```python
from build123d import *

# Parameters (mm, degrees)
F0_R           = 1.0414
F1_DEPTH       = 12.7
F3_D           = 2.0828
F3_CBORE_D     = 6.858
F3_CBORE_DEPTH = 4.1656


with BuildPart() as f1:
    # F0 (on Top) → F1 (new body)
    with BuildSketch(Plane.XY):
        with BuildLine():
            ThreePointArc((-68.834, -13.75156), (-68.090051, -15.547611), (-66.294, -16.29156))
            Line((-66.294, -16.29156), (66.294, -16.29156))
            ThreePointArc((66.294, -16.29156), (68.090051, -15.547611), (68.834, -13.75156))
            Line((68.834, -13.75156), (68.834, 13.75156))
            ThreePointArc((68.834, 13.75156), (68.090051, 15.547611), (66.294, 16.29156))
            Line((66.294, 16.29156), (-66.294, 16.29156))
            ThreePointArc((-66.294, 16.29156), (-68.090051, 15.547611), (-68.834, 13.75156))
            Line((-68.834, 13.75156), (-68.834, -13.75156))
        make_face()
        with Locations((-65.278, -10.16)):
            Circle(F0_R, mode=Mode.SUBTRACT)
        with Locations((65.278, -10.16)):
            Circle(F0_R, mode=Mode.SUBTRACT)
        with Locations((-65.278, 10.16)):
            Circle(F0_R, mode=Mode.SUBTRACT)
        with Locations((65.278, 10.16)):
            Circle(F0_R, mode=Mode.SUBTRACT)
    extrude(amount=F1_DEPTH)

    # F3 (through all)
    with Locations(Plane(origin=(0, 0, 0), x_dir=(1, 0, 0), z_dir=(0, 0, -1))):
        with Locations((-35.56, 5.08), (-35.56, -5.08)):
            CounterBoreHole(F3_D / 2, F3_CBORE_D / 2, F3_CBORE_DEPTH)


solid = f1.part
```
Could you check a few things on this model? Use its own coordinates, in mm. A direction names the side the tool comes from. Coordinates: 2 decimals unless noted, no trailing zeros. Write each loop counter-clockwise with the first axis right and the second up, starting at its lowest first coordinate (ties: lowest second). Pieces come first, ordered by that corner, then holes. Notation, with made-up numbers: (18, 77.5) - (36, 77.5) arc R8 cw to (36, 90.5) - close; hole circle Ø9 at (-34.5, -38.5). An arc over 180 degrees is marked (long way). Use a Markdown table: item, result.
Q1. Which directions (+Z, -Z, +X, -X, +Y, -Y) give clear straight access to the entire face, cutting with the end or side of a thin tool? Please do faces 1 (the cylindrical face through (68.07, -15.57, 6.26)), 2 (the flat face through (-35.6, -3.6, 4.166)).
Geometry check:
| item | result |
|---|---|
| face 1 | +Z, -Z, +X, -Y |
| face 2 | -Z |
Q2. Please list where these lines run through material, in increasing order: L1, parallel to Y at x = -35.56, z = 10.5; L2, parallel to X at y = -10, z = 8; L3, parallel to Y at x = -35.56, z = 1.9.
Geometry check:
| item | result |
|---|---|
| L1 | y = -16.29 to -6.12, -4.04 to 4.04, 6.12 to 16.29 |
| L2 | x = -68.83 to -66.31, -64.25 to 64.25, 66.31 to 68.83 |
| L3 | y = -16.29 to -8.51, -1.65 to 1.65, 8.51 to 16.29 |
Q3. I'm going to push flat-ended pins straight in: pin 1 Ø11 at (x, y) = (-35.56, -5.08) entering from -Z; pin 2 Ø1.9 at (x, y) = (65.278, -10.16) entering from +Z; pin 3 Ø2.5 at (x, y) = (-35.56, 5.08) entering from -Z. Where does each tip first touch, or does it pass through?
Geometry check:
| item | result |
|---|---|
| pin 1 | stops at z = 0 |
| pin 2 | passes through |
| pin 3 | stops at z = 4.17 |
Q4. Thinking about a two-plate mould opening in Y: for faces 3 (the flat face through (-1, -16.292, 6)), 4 (the flat face through (-35, 4, 4.166)), 5 (the flat face through (-1, 0, 12.7)), which applies, +Y half, -Y half, draft (parallel to the pull), parting line (faces both ways), or undercut?
Geometry check:
| item | result |
|---|---|
| face 3 | -Y half |
| face 4 | undercut |
| face 5 | draft |
Q5. Imagine slicing it at A-A (z = 2.5). List the corners of the cut face in (x, y) for me.
Geometry check:
| item | result |
|---|---|
| outline | (-68.83, -13.75) arc R2.54 ccw to (-66.29, -16.29) - (66.29, -16.29) arc R2.54 ccw to (68.83, -13.75) - (68.83, 13.75) arc R2.54 ccw to (66.29, 16.29) - (-66.29, 16.29) arc R2.54 ccw to (-68.83, 13.75) - close; hole circle Ø2.08 at (-65.28, -10.16); hole circle Ø2.08 at (-65.28, 10.16); hole circle Ø6.86 at (-35.56, -5.08); hole circle Ø6.86 at (-35.56, 5.08); hole circle Ø2.08 at (65.28, -10.16); hole circle Ø2.08 at (65.28, 10.16) |
